Work out the finished part from the listing and answer in its coordinate system (mm). A direction names the side the tool comes from. Give positions to 0.01 mm unless a question says otherwise; leave off trailing zeros. Order: outer loops, then holes, each group sorted by start corner. A loop starts at its lowest first (then second) coordinate and runs counter-clockwise, first axis right, second up. Notation, with made-up numbers: (-3.5, -12) - (1.5, -12) arc R20 ccw to (1.5, 4) - close; hole circle Ø6 at (-16, -28.75). An arc over 180 degrees is marked (long way). Put each result on its own line as item: value.
```python
from build123d import *

# Parameters (mm, degrees)
SKETCH1_W          = 73
SKETCH1_H          = 34
BASE_DEPTH         = 10
SKETCH3_W          = 70
SKETCH3_H          = 31
INSIDE_CUT_DEPTH   = 8.5
INSIDE_FILLET_R    = 5.5
OUTSIDE_FILLET_R   = 7
SKETCH4_W          = 16
SKETCH4_H          = 15
SCREW_SQUARE_DEPTH = 3
SCREW_FILLET_R     = 7.5
SKETCH5_R          = 4
CUT_EXTRUDE3_DEPTH = 3
SKETCH7_R          = 6.5
CUT_EXTRUDE4_DEPTH = 1.5


with BuildPart() as part:
    # Sketch1 → base (new body)
    with BuildSketch(Plane(origin=(0, 0, 0), x_dir=(1, 0, 0), z_dir=(0, 1, 0))):
        with Locations((3.513975155, -1.64052795)):
            Rectangle(SKETCH1_W, SKETCH1_H)
    extrude(amount=BASE_DEPTH)

    # Sketch3 → inside cut (cut)
    with BuildSketch(Plane.XZ):
        with Locations((3.513975155, 1.64052795)):
            Rectangle(SKETCH3_W, SKETCH3_H)
    extrude(amount=-INSIDE_CUT_DEPTH, mode=Mode.SUBTRACT)

    # inside fillet
    inside_fillet_edges = [part.edges().sort_by_distance(p)[0] for p in [
        (-31.486024845, 8.5, 1.64052795),
        (38.513975155, 8.5, 1.64052795),
    ]]
    fillet(inside_fillet_edges, radius=INSIDE_FILLET_R)

    # outside fillet
    outside_fillet_edges = [part.edges().sort_by_distance(p)[0] for p in [
        (40.013975155, 10, 1.64052795),
        (-32.986024845, 10, 1.64052795),
    ]]
    fillet(outside_fillet_edges, radius=OUTSIDE_FILLET_R)

    # Sketch4 → screw square (add)
    with BuildSketch(Plane.XZ):
        with Locations((48.013975155, 1.64052795)):
            Rectangle(SKETCH4_W, SKETCH4_H)
    extrude(amount=-SCREW_SQUARE_DEPTH)

    # screw fillet
    screw_fillet_edges = [part.edges().sort_by_distance(p)[0] for p in [
        (56.013975155, 1.5, -5.85947205),
        (56.013975155, 1.5, 9.14052795),
    ]]
    fillet(screw_fillet_edges, radius=SCREW_FILLET_R - 0.0001)  # a hair under: the kernel refuses the full size

    # Sketch5 → Cut-Extrude3 (cut)
    with BuildSketch(Plane(origin=(0, 3, 0), x_dir=(1, 0, 0), z_dir=(0, 1, 0))):
        with Locations(Location((47.513975155, -1.64052795, 0), (0, 0, 270))):
            Circle(SKETCH5_R)
    extrude(amount=-CUT_EXTRUDE3_DEPTH, mode=Mode.SUBTRACT)

    # Sketch7 → Cut-Extrude4 (cut)
    with BuildSketch(Plane(origin=(0, 3, 0), x_dir=(1, 0, 0), z_dir=(0, 1, 0))):
        with Locations(Location((47.513975155, -1.64052795, 0), (0, 0, 270))):
            Circle(SKETCH7_R)
    extrude(amount=-CUT_EXTRUDE4_DEPTH, mode=Mode.SUBTRACT)


solid = part.part
```
(1) Section D-D, the plane y = 4.75 is taken. Write down the section's boundary in (x, z).
Geometry check:
outline: (-32.76, -15.36) - (39.79, -15.36) - (39.79, 18.64) - (-32.76, 18.64) - close; hole (-31.2, -13.86) - (38.23, -13.86) - (38.23, 17.14) - (-31.2, 17.14) - close
(2) Section C-C, the plane x = 46 is taken. Write down the section's boundary in (y, z), then the cut area to 3 significant figures.
Geometry check:
outline: (0, -5.86) - (3, -5.86) - (3, -4.68) - (1.5, -4.68) - (1.5, -2.06) - (0, -2.06) - close; (0, 5.34) - (1.5, 5.34) - (1.5, 7.96) - (3, 7.96) - (3, 9.14) - (0, 9.14) - close
area: 14.9 mm²
(3) Determine the mould class of faces 1 (the face through (3, 5, 18.641)), 2 (the face through (38.018, 7.895, 1.403)), 3 (the face through (51.48, 0.76, 1.12)) for opening direction Z: pulls with the +Z half, pulls with the -Z half, needs draft (parallel to the pull), parting line crosses it, or undercut.
Geometry check:
face 1: pulls with the +Z half
face 2: needs draft
face 3: undercut
(4) A tool of negligible diameter and unlimited length cuts with its end or side. For faces 4 (the face through (43, 1.5, 2)), 5 (the face through (-29.918, 6.846, 1.858)), 6 (the face through (44, 1, 9.141)), from which of +Z, -Z, +X, -X, +Y, -Y can it reach the whole face along a straight path? Write none if from no direction.
Geometry check:
face 4: +Y
face 5: -Y
face 6: +Z, +X, +Y, -Y
(5) Given pin 1 (10.5 mm diameter, centred on x = 47.51, z = 1.64, fed in from +Y); pin 2 (10.5 mm diameter, centred on x = 47.5, z = 4.5, fed in from +Y); pin 3 (3.5 mm diameter, centred on x = 44.5, y = 2, fed in from +Z), each flat-ended and moving along its own axis, determine where each tip first touches the part or whether it passes through.
Geometry check:
pin 1: stops at y = 1.5
pin 2: stops at y = 3
pin 3: stops at z = 9.14
(6) Section A-A, the plane x = 10 is taken. Write down the section's boundary in (y, z), then the cut area to 3 significant figures.
Geometry check:
outline: (0, -15.36) - (10, -15.36) - (10, 18.64) - (0, 18.64) - (0, 17.14) - (8.5, 17.14) - (8.5, -13.86) - (0, -13.86) - close
area: 76.5 mm²
(7) Straight lines are drawn through the part: line 1 (X direction, y = 2, z = -7.5); line 2 (Z direction, x = -21.5, y = 4); line 3 (Y direction, x = -2, z = 10). For each, find the intervals that lie inside material, in ascending order.
Geometry check:
line 1: x = -32.99 to -31.49, 38.51 to 40.01
line 2: z = -15.36 to -13.86, 17.14 to 18.64
line 3: y = 8.5 to 10
(8) Section B-B, the plane z = -8 is taken. Write down the section's boundary in (x, y).
Geometry check:
outline: (-32.99, 0) - (-31.49, 0) - (-31.49, 3) arc R5.5 cw to (-25.99, 8.5) - (33.01, 8.5) arc R5.5 cw to (38.51, 3) - (38.51, 0) - (40.01, 0) - (40.01, 3) arc R7 ccw to (33.01, 10) - (-25.99, 10) arc R7 ccw to (-32.99, 3) - close
